```python
from build123d import *

# Parameters (mm, degrees)
SKETCH1_W               = 11.5
SKETCH1_H               = 15.75
SKETCH2_R               = 6
BOSS_EXTRUDE1_DEPTH     = 6
SKETCH3_R               = 3
BOSS_EXTRUDE2_DEPTH     = 12
SKETCH4_R               = 1.6
CUT_EXTRUDE1_DEPTH      = 6
CUT_EXTRUDE2_DEPTH      = 94.60659699
CUT_EXTRUDE2_DEPTH_BACK = 12


with BuildPart() as part:
    # Sketch1 → Revolve1 (revolve)
    with BuildSketch(Plane(origin=(0, 0, 0), x_dir=(0, 0, -1), z_dir=(1, 0, 0)), mode=Mode.PRIVATE) as revolve1_sk:
        with Locations((35.75, -25.375)):
            Rectangle(SKETCH1_W, SKETCH1_H)
        Polygon((30, -17.5), (0, -17.5), (0, -35), (30, -35), (30, -33.25), align=None)
        Polygon((0, -17.5), (-25, -17.5), (-25, -35.85), (0, -35.85), (0, -35), align=None)
    revolve(revolve1_sk.sketch.rotate(Axis((0, -17.5, 25), (0, 0, -1)), 270), axis=Axis((0, -17.5, 25), (0, 0, -1)))

    # Sketch2 → Boss-Extrude1 (add)
    with BuildSketch(Plane.XY.offset(25)):
        with Locations(Location((0, -10.5, 0), (0, 0, 180))):
            Circle(SKETCH2_R)
    extrude(amount=BOSS_EXTRUDE1_DEPTH)

    # Sketch3 → Boss-Extrude2 (add)
    with BuildSketch(Plane.XY.offset(31)):
        with Locations((0, -10.5)):
            Circle(SKETCH3_R)
    extrude(amount=BOSS_EXTRUDE2_DEPTH)

    # Sketch4 → Cut-Extrude1 (cut)
    with BuildSketch(Plane.XY.offset(25)):
        with Locations((-15.5, -17.5)):
            Circle(SKETCH4_R)
        with Locations((15.5, -17.5)):
            Circle(SKETCH4_R)
        with Locations((-7.75, -4.076606241)):
            Circle(SKETCH4_R)
        with Locations((7.75, -4.076606241)):
            Circle(SKETCH4_R)
        with Locations((7.75, -30.923393759)):
            Circle(SKETCH4_R)
        with Locations((-7.75, -30.923393759)):
            Circle(SKETCH4_R)
    extrude(amount=-CUT_EXTRUDE1_DEPTH, mode=Mode.SUBTRACT)

    # Sketch5 → Cut-Extrude2 (cut, two sides: drawn at the far end of the back side and taken through both)
    with BuildSketch(Plane.XY.offset(43).offset(-CUT_EXTRUDE2_DEPTH_BACK)):
        with BuildLine():
            Line((-1.658312395, -8), (1.658312395, -8))
            ThreePointArc((1.658312395, -8), (0, -7.5), (-1.658312395, -8))
        make_face()
    extrude(amount=CUT_EXTRUDE2_DEPTH + CUT_EXTRUDE2_DEPTH_BACK, mode=Mode.SUBTRACT)


solid = part.part
```
Verification items for the finished model (mm, model axes). A direction names the side the tool comes from. Coordinates: 2 decimals unless noted, no trailing zeros. Loops run counter-clockwise (first coordinate to the right, second up) from the corner with the lowest first, then second, coordinate; pieces in that order, holes last. Notation, with made-up numbers: (-23, 83) -> (-18, 83) arc R16 cw to (-18, 87) -> close; hole circle Ø2 at (89.5, -27.75). An arc over 180 degrees is marked (long way). Answer in a Markdown table with one row per item. Add a question column.
1. Draft check along Y on faces 1 (the face through (14.32, -16.42, 22.04)), 2 (the face through (0, -11, 43)), 3 (the face through (1.301, -4.643, 27.958)), 4 (the face through (0, -8, 37)). Enter one of: +Y half, -Y half, draft (parallel to the pull), parting line (faces both ways), or undercut.
2. Material ranges on probe 1 along X at (y, z) = (-17, 21); probe 2 along Y at (x, z) = (7, 21); probe 3 along Z at (x, y) = (-12, -31), recorded low to high. Write a range as [from, to].
3. Access from +Z, -Z, +X, -X, +Y, -Y to the whole of each face (thin tool, end or side, straight path). Record for faces 5 (the face through (-8, -31, 19)), 6 (the face through (-2.389, -35.694, 12.325)), 7 (the face through (-2.28, -34.85, -15.21)).
4. Section check B-B, the plane x = 7.75. Enter the section's corners in (y, z), then the cut area to 3 significant figures.
5. Section check C-C, the plane z = -35.5. Enter the section's corners in (x, y), then the cut area to 3 significant figures.
6. Section check D-D, the plane y = -28. Enter the section's corners in (x, z), then the cut area to 3 significant figures.
7. Depth check by flat-ended pin: P1, Ø3.5, axis at x = -0.5, z = 39.5, coming from the +Y side; P2, Ø1.9, axis at x = -7.75, y = -30.92, coming from the +Z side; P3, Ø4, axis at y = -8, z = 18.5, coming from the -X side; P4, Ø1, axis at y = -15.5, z = 33.5, coming from the -X side. Enter the tip coordinate at first touch or a pass-through.
8. Section check A-A, the plane y = -17.5. Enter the section's corners in (x, z), then the cut area to 3 significant figures.
Derived:
| question | item | result |
|---|---|---|
| 1 | face 1 | undercut |
| 1 | face 2 | draft |
| 1 | face 3 | parting line |
| 1 | face 4 | +Y half |
| 2 | probe 1 | x = [-18.34, -17.02], [-13.98, 13.98], [17.02, 18.34] |
| 2 | probe 2 | y = [-34.46, -32.34], [-29.51, -5.49], [-2.66, -0.54] |
| 2 | probe 3 | z = [0, 25] |
| 3 | face 5 | +Z |
| 3 | face 6 | +Z, -Z |
| 3 | face 7 | -Z |
| 4 | outline | (-34.13, 0) -> (-33.19, 0) -> (-33.19, -30) -> (-31.21, -30) -> (-31.21, -41.5) -> (-3.79, -41.5) -> (-3.79, -30) -> (-1.81, -30) -> (-1.81, 0) -> (-0.87, 0) -> (-0.87, 25) -> (-2.48, 25) -> (-2.48, 19) -> (-5.68, 19) -> (-5.68, 25) -> (-29.32, 25) -> (-29.32, 19) -> (-32.52, 19) -> (-32.52, 25) -> (-34.13, 25) -> close |
| 4 | area | 2,050 mm² |
| 5 | outline | circle Ø31.5 at (0, -17.5) |
| 5 | area | 779 mm² |
| 6 | outline | (-15.05, 0) -> (-14, 0) -> (-14, -30) -> (-11.74, -30) -> (-11.74, -41.5) -> (11.74, -41.5) -> (11.74, -30) -> (14, -30) -> (14, 0) -> (15.05, 0) -> (15.05, 25) -> (-15.05, 25) -> close |
| 6 | area | 1,860 mm² |
| 7 | P1 | stops at y = -8 |
| 7 | P2 | stops at z = 19 |
| 7 | P3 | stops at x = -16.75 |
| 7 | P4 | passes through |
| 8 | outline | (-18.35, 0) -> (-17.5, 0) -> (-17.5, -30) -> (-15.75, -30) -> (-15.75, -41.5) -> (15.75, -41.5) -> (15.75, -30) -> (17.5, -30) -> (17.5, 0) -> (18.35, 0) -> (18.35, 25) -> (17.1, 25) -> (17.1, 19) -> (13.9, 19) -> (13.9, 25) -> (-13.9, 25) -> (-13.9, 19) -> (-17.1, 19) -> (-17.1, 25) -> (-18.35, 25) -> close |
| 8 | area | 2,290 mm² |
